The model under review builds one solid part; all positions refer to its coordinate system, in mm. A direction names the side the tool comes from. Round coordinates to 2 decimals unless told otherwise and drop trailing zeros. Write each loop counter-clockwise with the first axis right and the second up, starting at its lowest first coordinate (ties: lowest second). Pieces come first, ordered by that corner, then holes. Notation, with made-up numbers: M -38,46.25 L -11,46.25 A25 cw -11,71.25 Z; hole C 56,38.25 d11. An arc over 180 degrees is marked long. One line per item, written item: value. Start each with the question number.
1) For P1, Ø1.2, axis at x = 0, y = 2.5, coming from the -Z side; P2, Ø0.6, axis at y = -3, z = 5.5, coming from the -X side; P3, Ø1.1, axis at x = 0, z = 7.5, coming from the -Y side, all flat-tipped, find the tip position at first contact; note any pin that passes through.
2) Take a section at B-B, the plane y = 1. Write out the cut boundary in (x, z), and give its area (3 significant figures).
3) Take a section at C-C, the plane x = 2.1. Write out the cut boundary in (y, z), and give its area (3 significant figures).
4) Mouldability with a two-part tool opening along Y and no side actions: class faces 1 (the face through (1.42, 3.72, 6.29)), 2 (the face through (-2.5, -1, 2)), 3 (the face through (0.28, -1.23, -1.07)) as +Y half, -Y half, draft (parallel to the pull), parting line (faces both ways), or undercut.
5) Wall thickness on probe 1 along Y at (x, z) = (0.05, 1.25); probe 2 along Y at (x, z) = (0, 4.95); probe 3 along Z at (x, y) = (-1.9, -2): over which ranges is each line inside the solid? List them lowest first.
6) Tool access review of faces 4 (the face through (-0.13, 3.49, 6.37)), 5 (the face through (1.503, 1.41, 6.288)), 6 (the face through (-1.487, 1.361, 6.288)), 7 (the face through (0.268, -1.853, -0.219)): name each direction out of +Z, -Z, +X, -X, +Y, -Y from which nothing blocks a thin tool from reaching the whole face with its end or side.
7) Take a section at A-A, the plane z = 7.75. Write out the cut boundary in (x, y).
Autodesk Inventor part; units mm, degrees
ref_plane "YZ Plane" through (0, 0, 0) normal (1, 0, 0) x (0, 1, 0)
ref_plane "XZ Plane" through (0, 0, 0) normal (0, 1, 0) x (-1, 0, 0)
ref_plane "XY Plane" through (0, 0, 0) normal (0, 0, 1) x (1, 0, 0)
sketch "Skizze1" plane through (0, 0, 0) normal (0, 0, 1) x (1, 0, 0)
  line L0 (-2.6, -5.1) -> (2.6, -5.1)
  line L1 (2.6, -5.1) -> (2.6, 3.2)
  line L2 (-2.6, -5.1) -> (-2.6, 3.2)
  line L3 (-1.3, 5.1) -> (1.3, 5.1)
  line L4 (0, -5.1) -> (0, 5.1) construction
  line L5 (-2.6, 3.2) -> (-1.3, 5.1)
  line L6 (1.3, 5.1) -> (2.6, 3.2)
  point P0 (0, 0)
  point P1 (0, 0)
  dimension "d0" = 5.2
  dimension "d1" = 8.3
  dimension "d2" = 2.6
  dimension "d3" = 10.2
extrude "Extrusion1" add sketch "Skizze1" along normal blind 3.33
sketch "Skizze3" plane through (0, 0, 3.33) normal (0, 0, 1) x (1, 0, 0)
  line L0 (0, -0.674) -> (0, 0.674) construction
  line L1 (0, 0) -> (0, 4.35) construction
  line L2 (-0.989, 4.35) -> (0.989, 4.35)
  line L3 (0.989, 4.35) -> (1.8672, 3.0665)
  line L4 (-0.989, 4.35) -> (-1.8885, 3.0353)
  line L5 (-1.3, 5.1) -> (-2.6, 3.2)
  line L6 (2.6, 3.2) -> (1.3, 5.1)
  circle A0 centre (0, 2.5) radius 0.5 construction
  circle A1 centre (0, 2.5) radius 0.5 construction
  line L7 (-1.8885, 3.0353) -> (-1.8885, 2.5219)
  line L8 (1.8672, 3.0665) -> (1.8672, 2.5531)
  arc A2 (-1.8885, 2.5219) -> (1.8672, 2.5531) centre (-0.0105, 2.5219) ccw
  dimension "d11" = 1.348
  dimension "d12" = 4.35
  dimension "d13" = 1.978
extrude "Extrusion3" add sketch "Skizze3" along normal blind 6
sketch "Skizze4" plane through (0, 0, 3.33) normal (0, 0, 1) x (1, 0, 0)
  line L0 (-2.6, 3.2) -> (-2.6, -5.1) construction
  line L1 (-2.6, -4.6629) -> (-2.6, -0.9339) construction
  line L2 (-1.8645, -4.35) -> (1.8645, -4.35)
  arc A0 (-1.8885, 2.5219) -> (1.8672, 2.5531) centre (-0.0105, 2.5219) ccw
  line L3 (-1.8645, -4.35) -> (-1.8645, -2.5085)
  line L4 (1.8645, -4.35) -> (1.8645, -2.5085)
  arc A1 (1.8645, -2.5085) -> (-1.8645, -2.5085) centre (0, -2.5085) ccw
  line L5 (-0.4867, 0.8046) -> (0.4867, 0.8046)
  line L6 (0.4867, 0.8046) -> (0.4867, -0.8046)
  line L7 (0.4867, -0.8046) -> (-0.4867, -0.8046)
  line L8 (-0.4867, -0.8046) -> (-0.4867, 0.8046)
  line L9 (-0.4867, 0.8046) -> (0.4867, -0.8046) construction
  point P0 (0, 0)
  point P1 (0, 0)
  dimension "d18" = 3.729
extrude "Extrusion4" add sketch "Skizze4" along normal blind 6
sketch "Skizze5" plane through (0, 0, 9.33) normal (0, 0, 1) x (1, 0, 0)
  line L0 (0, -2.5) -> (0, 2.5) construction
  circle A0 centre (0, 2.5) radius 1
  circle A1 centre (0, -2.5) radius 1
  point P0 (0, 0)
  point P1 (0, 0)
  point P2 (0, 0)
  dimension "d22" = 5
  dimension "d23" = 2
  dimension "d24" = 2
extrude "Extrusion5" cut sketch "Skizze5" against normal blind 6
sketch "Skizze6" plane through (2.6, -5.1, 0) normal (1, 0, 0) x (0, 0, -1)
  line L0 (-3.33, 4.3914) -> (-9.33, 4.3914) construction
  line L1 (-3.33, 4.3914) -> (-2.88, 4.3914) construction
  line L2 (0, 5.1) -> (-0.45, 5.1) construction
  line L3 (0, 0) -> (-3.33, 0)
  line L4 (0, 8.3) -> (-3.33, 8.3)
  line L5 (-2.88, 0) -> (-0.45, 0)
  line L6 (-0.45, 0) -> (-0.45, 8.3)
  line L7 (-0.45, 8.3) -> (-2.88, 8.3)
  line L8 (-2.88, 8.3) -> (-2.88, 0)
  dimension "d31" = 0.45
  dimension "d32" = 0.45
extrude "Extrusion6" cut sketch "Skizze6" against normal blind 0.1
sketch "Skizze7" plane through (1.3, 5.1, 3.33) normal (0.8253, 0.5647, 0) x (0, 0, -1)
  line L0 (0.45, -2.3022) -> (0, -2.3022)
  line L1 (3.33, 0) -> (0, 0)
  line L2 (0.45, -2.3022) -> (2.8887, -2.3022)
  line L3 (2.8887, -2.3022) -> (2.8887, 0)
  line L4 (2.8887, 0) -> (0.45, 0)
  line L5 (0.45, 0) -> (0.45, -2.3022)
  point P0 (3.33, -3.475)
extrude "Extrusion7" cut sketch "Skizze7" against normal blind 0.1
sketch "Skizze8" plane through (-1.3, 5.1, 0) normal (0, 1, 0) x (1, 0, 0)
  line L0 (2.6, -2.88) -> (2.6, -3.33)
  line L1 (0, 0) -> (0, -3.33)
  line L2 (2.6, -2.88) -> (0, -2.88)
  line L3 (0, -2.88) -> (0, -0.4356)
  line L4 (0, -0.4356) -> (2.6, -0.4356)
  line L5 (2.6, -0.4356) -> (2.6, -2.88)
  point P0 (1.3, 0)
extrude "Extrusion8" cut sketch "Skizze8" against normal blind 0.1
sketch "Skizze9" plane through (-2.6, 3.2, 0) normal (-0.8253, 0.5647, 0) x (0, 0, 1)
  line L0 (2.88, 3.7704) -> (2.88, 2.3022)
  line L1 (0, 0) -> (3.33, 0)
  line L2 (2.88, 2.3022) -> (0.436, 2.3022)
  line L3 (0.436, 2.3022) -> (0.436, 0)
  line L4 (0.436, 0) -> (2.88, 0)
  line L5 (2.88, 0) -> (2.88, 2.3022)
  point P0 (0, -1.1728)
  dimension "d39" = 2.444
extrude "Extrusion9" cut sketch "Skizze9" against normal blind 0.1
sketch "Skizze10" plane through (-2.6, -5.1, 0) normal (-1, 0, 0) x (0, 0, 1)
  line L0 (0.4366, 8.3229) -> (2.8806, 8.3229)
  line L1 (2.8806, 8.3229) -> (2.8806, 0)
  line L2 (2.8806, 0) -> (0.4366, 0)
  line L3 (0.4366, 0) -> (0.4366, 8.3229)
  point P0 (0, 5.1)
  dimension "d42" = 2.444
extrude "Extrusion10" cut sketch "Skizze10" against normal blind 0.1
sketch "Skizze11" plane through (-2.6, -5.1, 0) normal (0, -1, 0) x (1, 0, 0)
  line L0 (1.3, 2.88) -> (0.0157, 2.88)
  line L1 (3.8473, 0.4413) -> (5.1175, 0.4413)
  line L2 (0.0989, 2.88) -> (5.1175, 2.88)
  line L3 (5.1175, 2.88) -> (5.1175, 0.4413)
  line L4 (5.1175, 0.4413) -> (0.0989, 0.4413)
  line L5 (0.0989, 0.4413) -> (0.0989, 2.88)
  point P0 (2.6, 0)
extrude "Extrusion11" cut sketch "Skizze11" against normal blind 0.1
sketch "Skizze12" plane through (0, 0, 0) normal (0, 0, -1) x (-1, 0, 0)
  circle A0 centre (0, -2.5) radius 1 construction
  circle A1 centre (0, -2.5) radius 1 construction
  circle A2 centre (0, 2.5) radius 1 construction
  circle A3 centre (0, 2.5) radius 1 construction
  circle A4 centre (0, -2.5) radius 1.3
  circle A5 centre (0, 2.5) radius 1.3
  point P0 (0, 0)
  dimension "d47" = 2.6
extrude "Extrusion12" add sketch "Skizze12" along normal blind 3
chamfer "Fase1" distance 0.2 angle 45 2 edges at (1.3, -2.5, -3) (1.3, 2.5, -3)
sketch "Skizze13" plane through (0, -2.5, -3) normal (0, 0, -1) x (-1, 0, 0)
  circle A0 centre (0, 0) radius 1.1
  circle A1 centre (0, 5) radius 1.1
  point P0 (0, 2.5)
hole "Bohrung1" at (0, 2.5, -3) at (0, -2.5, -3) direction (0, 0, 1) diameter 1.4 depth 4.5 tip angle 118
sketch "Skizze14" plane through (0, -2.5, -3) normal (0, 0, -1) x (-1, 0, 0)
  circle A0 centre (0, 0) radius 1.3 construction
  circle A1 centre (0, 5) radius 1.3 construction
  line L0 (2.6, -2.6) -> (-2.6, -2.6) construction
  line L1 (2.6, 5.7) -> (2.6, -2.6) construction
  line L2 (1.3, 7.6) -> (2.6, 5.7) construction
  line L3 (-1.3, 7.6) -> (1.3, 7.6) construction
  line L4 (-2.6, 5.7) -> (-1.3, 7.6) construction
  line L5 (-2.6, -2.6) -> (-2.6, 5.7) construction
  line L6 (-1.3, 0) -> (1.3, 0)
  line L7 (-1.3, 5) -> (1.3, 5)
  circle A2 centre (0, 0) radius 1.3
  arc A3 (-1.3, 0) -> (1.3, 0) centre (0, 0) ccw
  circle A4 centre (0, 5) radius 0.7
  arc A5 (1.3, 5) -> (-1.3, 5) centre (0, 5) ccw
  point P0 (0, 2.5)
extrude "Extrusion13" cut sketch "Skizze14" against normal blind 2.5 contours L6 A2 | A4 L7 A5 | L7 A4 picked at (-0.4207, -0.1037) picked at (0.2266, 5.0558)
properties part number "stecker2"
Checked values:
1. P1: stops at z = 1.56
1. P2: stops at x = -1.86
1. P3: stops at y = -4.35
2. outline: M -2.6,0 L 2.6,0 L 2.6,0.45 L 2.5,0.45 L 2.5,2.88 L 2.6,2.88 L 2.6,3.33 L 1.09,3.33 L 1.09,9.33 L -1.11,9.33 L -1.11,3.33 L -2.6,3.33 L -2.6,2.88 L -2.5,2.88 L -2.5,0.44 L -2.6,0.44 Z
2. area: 30.0 mm2
3. outline: M -5.1,0 L 3.93,0 L 3.93,0.44 L 3.75,0.44 L 3.75,2.88 L 3.93,2.88 L 3.93,3.33 L -5.1,3.33 L -5.1,2.88 L -5,2.88 L -5,0.44 L -5.1,0.44 Z
3. area: 29.4 mm2
4. face 1: +Y half
4. face 2: draft
4. face 3: undercut
5. probe 1: y = -5 to -3.2, -1.8 to 1.8, 3.2 to 5
5. probe 2: y = -4.35 to -3.5, -1.5 to 1.5, 3.5 to 4.35
5. probe 3: z = 0 to 3.33
6. face 4: +Z
6. face 5: +Z, +X
6. face 6: +Z, -X
6. face 7: -Z
7. outline: M -1.89,2.52 A1.88 ccw -0.49,0.71 L -0.49,-0.71 A1.86 ccw -1.86,-2.51 L -1.86,-4.35 L 1.86,-4.35 L 1.86,-2.51 A1.86 ccw 0.49,-0.71 L 0.49,0.71 A1.88 ccw 1.87,2.55 L 1.87,3.07 L 0.99,4.35 L -0.99,4.35 L -1.89,3.04 Z; hole C 0,-2.5 d2; hole C 0,2.5 d2
